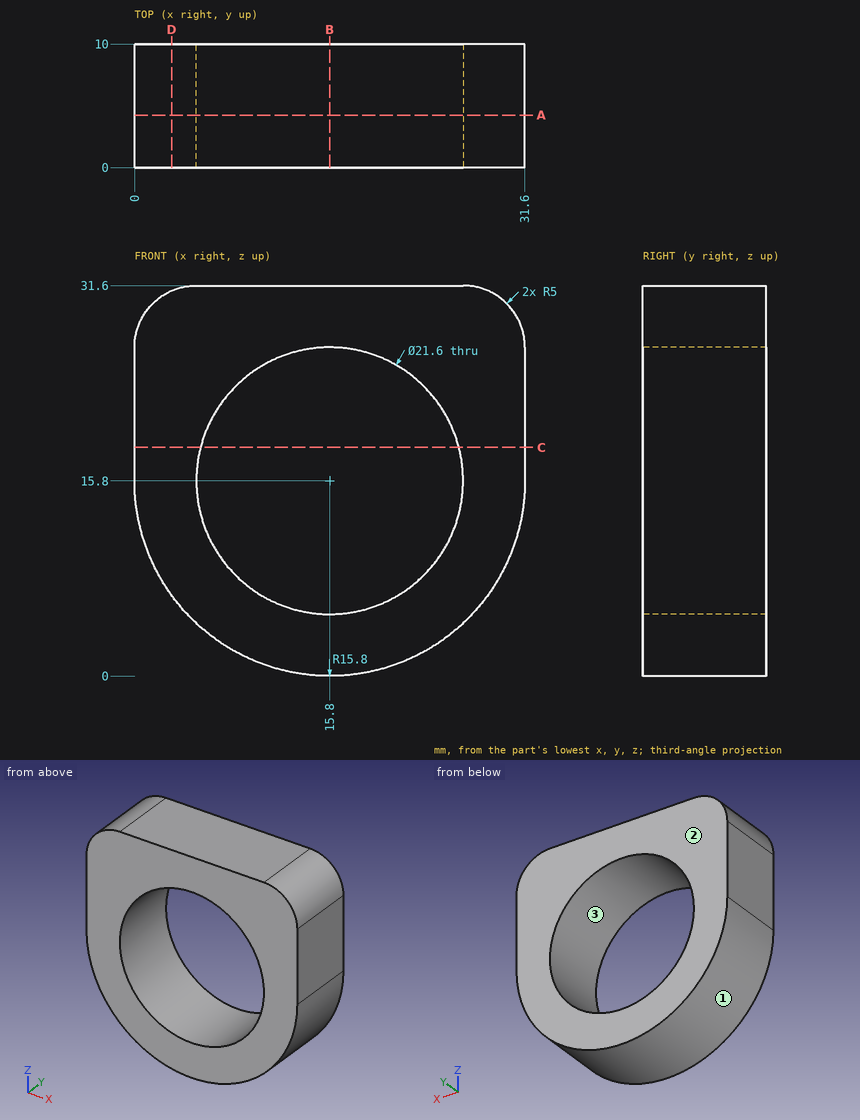
Input: dimensioned drawing with shaded views. Units: mm. Origin: part minimum x, y, z. Give positions to 0.01 mm unless a question says otherwise; leave off trailing zeros. Write each loop counter-clockwise with the first axis right and the second up, starting at its lowest first coordinate (ties: lowest second). Pieces come first, ordered by that corner, then holes.
1. Pull-direction query (X, two-part tool) for the marked faces 1, 2 and 3; classes: +X half, -X half, draft (parallel to the pull), parting line (faces both ways), or undercut.
2. Material intervals for line 1 along X through (y, z) = (6.25, 15.8); line 2 along Z through (x, y) = (7.5, 9.25), sorted ascending.
3. Section query D-D (x = 3). Return the cut outline in (y, z).
4. First-contact query: pin 1 (1.5 mm diameter, centred on y = 4.5, z = 13.5, fed in from -X); pin 2 (2 mm diameter, centred on x = 3.5, y = 5.5, fed in from -Z). Flat tips, straight axial feed; report the tip coordinate or a pass-through.
5. Section query B-B (x = 15.8). Return the cut outline in (y, z), then the cut area to 4 significant figures.
6. Section query C-C (z = 18.5). Return the cut outline in (x, y).
7. Section query A-A (y = 4.25). Return the cut outline in (x, z).
Output values:
1. face 1: parting line
1. face 2: draft
1. face 3: undercut
2. line 1: x = 0 to 5, 26.6 to 31.6
2. line 2: z = 2.36 to 8.89, 22.71 to 31.6
3. outline: (0, 6.54) - (10, 6.54) - (10, 31.18) - (0, 31.18) - close
4. pin 1: stops at x = 0.08
4. pin 2: stops at z = 4.76
5. outline: (0, 0) - (10, 0) - (10, 5) - (0, 5) - close; (0, 26.6) - (10, 26.6) - (10, 31.6) - (0, 31.6) - close
5. area: 100.0 mm2
6. outline: (0, 0) - (5.34, 0) - (5.34, 10) - (0, 10) - close; (26.26, 0) - (31.6, 0) - (31.6, 10) - (26.26, 10) - close
7. outline: (0, 15.8) arc R15.8 ccw to (31.6, 15.8) - (31.6, 26.6) arc R5 ccw to (26.6, 31.6) - (5, 31.6) arc R5 ccw to (0, 26.6) - close; hole circle Ø21.6 at (15.8, 15.8)
